from build123d import *

# Parameters (mm, degrees)
SKETCH1_R           = 3.429
SKETCH1_R_2         = 2.54
BOSS_EXTRUDE1_DEPTH = 3.2004
SKETCH2_R           = 2.413
CUT_EXTRUDE1_DEPTH  = 3.2004
SKETCH5_R           = 1.7272
SKETCH5_W           = 40.894
SKETCH5_H           = 20.32
CUT_EXTRUDE3_DEPTH  = 203.721029268
CUT_EXTRUDE5_DEPTH  = 3.2004
SKETCH6_R           = 2.54
CUT_EXTRUDE4_DEPTH  = 203.721029268
SKETCH9_R           = 2.159
CUT_EXTRUDE6_DEPTH  = 3.2004
SKETCH10_W          = 107.95
SKETCH10_H          = 3.2512
CUT_EXTRUDE7_DEPTH  = 3.2004
SKETCH11_R          = 3.429
SKETCH11_R_2        = 2.54
CUT_EXTRUDE8_DEPTH  = 3.2004
CUT_EXTRUDE9_DEPTH  = 3.2004
SKETCH15_R          = 2.159
CUT_EXTRUDE10_DEPTH = 3.2004
BOSS_EXTRUDE2_DEPTH = 3.2004
FILLET1_R           = 5.08
CUT_EXTRUDE11_DEPTH = 3.2004
CUT_EXTRUDE12_DEPTH = 3.2004
FILLET3_R           = 5.08


with BuildPart() as part:
    # Sketch1 → Boss-Extrude1 (new body)
    with BuildSketch(Plane.XY):
        with BuildLine():
            Line((0, 0), (120.015, 0))
            ThreePointArc((120.015, 0), (130.351788396, 3.075697789), (137.325636158, 11.302152592))
            Line((137.325636158, 11.302152592), (155.2575, 52.11572))
            ThreePointArc((155.2575, 52.11572), (157.54731739, 67.602183396), (151.630955452, 82.09599151))
            ThreePointArc((151.630955452, 82.09599151), (60.0075, 127.266502568), (-31.615955452, 82.09599151))
            ThreePointArc((-31.615955452, 82.09599151), (-37.53231739, 67.602183396), (-35.2425, 52.11572))
            Line((-35.2425, 52.11572), (-17.310636158, 11.302152592))
            ThreePointArc((-17.310636158, 11.302152592), (-10.336788396, 3.075697789), (0, 0))
        make_face()
        with Locations((120.015, 18.90776)):
            Circle(SKETCH1_R, mode=Mode.SUBTRACT)
        with Locations((0, 18.90776)):
            Circle(SKETCH1_R_2, mode=Mode.SUBTRACT)
        with Locations((19.734727626, 25.566426992)):
            Circle(SKETCH1_R_2, mode=Mode.SUBTRACT)
    extrude(amount=BOSS_EXTRUDE1_DEPTH)

    # Sketch2 → Cut-Extrude1 (cut)
    with BuildSketch(Plane(origin=(0, 0, 0), x_dir=(-1, 0, 0), z_dir=(0, 0, -1))):
        with Locations((-92.0115, 52.11572)):
            Circle(SKETCH2_R)
        with Locations((-76.0095, 52.11572)):
            Circle(SKETCH2_R)
        with Locations((-44.0055, 52.11572)):
            Circle(SKETCH2_R)
        with Locations((-28.0035, 52.11572)):
            Circle(SKETCH2_R)
    extrude(amount=-CUT_EXTRUDE1_DEPTH, mode=Mode.SUBTRACT)

    # Sketch5 → Cut-Extrude3 (cut, through all)
    with BuildSketch(Plane(origin=(0, 0, 0), x_dir=(-1, 0, 0), z_dir=(0, 0, -1))):
        with Locations((-98.932021353, 23.907759967)):
            Circle(SKETCH5_R)
        with Locations((-48.432021353, 13.907760033)):
            Circle(SKETCH5_R)
        with Locations((-48.432021353, 23.907759967)):
            Circle(SKETCH5_R)
        with Locations((-98.932021353, 13.907760033)):
            Circle(SKETCH5_R)
        with Locations((-73.682021353, 18.90776)):
            Rectangle(SKETCH5_W, SKETCH5_H)
    extrude(amount=-CUT_EXTRUDE3_DEPTH, mode=Mode.SUBTRACT)

    # Sketch7 → Cut-Extrude5 (cut)
    with BuildSketch(Plane(origin=(0, 0, 0), x_dir=(-1, 0, 0), z_dir=(0, 0, -1))):
        with BuildLine():
            Line((-98.193021353, 19.92376), (-94.129021353, 19.92376))
            Line((-94.129021353, 19.92376), (-94.129021353, 17.89176))
            Line((-94.129021353, 17.89176), (-98.193021353, 17.89176))
            ThreePointArc((-98.193021353, 17.89176), (-99.209021353, 18.90776), (-98.193021353, 19.92376))
        make_face()
        with BuildLine():
            Line((-53.235021353, 19.92376), (-49.171021353, 19.92376))
            ThreePointArc((-49.171021353, 19.92376), (-48.155021353, 18.90776), (-49.171021353, 17.89176))
            Line((-49.171021353, 17.89176), (-53.235021353, 17.89176))
            Line((-53.235021353, 17.89176), (-53.235021353, 19.92376))
        make_face()
    extrude(amount=-CUT_EXTRUDE5_DEPTH, mode=Mode.SUBTRACT)

    # Sketch6 → Cut-Extrude4 (cut, through all)
    with BuildSketch(Plane(origin=(0, 0, 0), x_dir=(-1, 0, 0), z_dir=(0, 0, -1))):
        with Locations((-99.400822485, 30.809360937)):
            Circle(SKETCH6_R)
    extrude(amount=-CUT_EXTRUDE4_DEPTH, mode=Mode.SUBTRACT)

    # Sketch9 → Cut-Extrude6 (cut)
    with BuildSketch(Plane.XY.offset(3.2004)):
        with Locations((21.9075, 3.81)):
            Circle(SKETCH9_R)
        with Locations((60.0075, 3.81)):
            Circle(SKETCH9_R)
        with Locations((98.1075, 3.81)):
            Circle(SKETCH9_R)
    extrude(amount=-CUT_EXTRUDE6_DEPTH, mode=Mode.SUBTRACT)

    # Sketch10 → Cut-Extrude7 (cut)
    with BuildSketch(Plane.XY.offset(3.2004)):
        with Locations((60.0075, 46.68012)):
            Rectangle(SKETCH10_W, SKETCH10_H)
    extrude(amount=-CUT_EXTRUDE7_DEPTH, mode=Mode.SUBTRACT)

    # Sketch11 → Cut-Extrude8 (cut)
    with BuildSketch(Plane.XY.offset(3.2004)):
        with Locations((126.474462556, 80.535782848)):
            Circle(SKETCH11_R)
        with Locations((105.860285087, 92.437383759)):
            Circle(SKETCH11_R_2)
    extrude(amount=-CUT_EXTRUDE8_DEPTH, mode=Mode.SUBTRACT)

    # Sketch14 → Cut-Extrude9 (cut)
    with BuildSketch(Plane(origin=(0, 0, 0), x_dir=(-1, 0, 0), z_dir=(0, 0, -1))):
        with BuildLine():
            Line((-44.300963253, 126.193661773), (-33.172711709, 93.735154568))
            Line((-33.172711709, 93.735154568), (17.974883496, 60.568226691))
            Line((17.974883496, 60.568226691), (31.788532543, 81.870619617))
            ThreePointArc((31.788532543, 81.870619617), (-1.866863458, 111.567353903), (-44.300963253, 126.193661773))
        make_face()
    extrude(amount=-CUT_EXTRUDE9_DEPTH, mode=Mode.SUBTRACT)

    # Sketch15 → Cut-Extrude10 (cut)
    with BuildSketch(Plane.XY.offset(3.2004)):
        with Locations((8.255, 18.90776)):
            Circle(SKETCH15_R)
        with Locations((107.05592, 18.90776)):
            Circle(SKETCH15_R)
    extrude(amount=-CUT_EXTRUDE10_DEPTH, mode=Mode.SUBTRACT)

    # Sketch16 → Boss-Extrude2 (add)
    with BuildSketch(Plane.XY.offset(3.2004)):
        with BuildLine():
            Line((-45.041102147, 54.757414103), (-19.827237301, 11.4051976))
            ThreePointArc((-19.827237301, 11.4051976), (-11.436759498, 3.05471175), (0, 0))
            ThreePointArc((0, 0), (-10.916945649, 29.711492853), (-17.974883496, 60.568226691))
            Line((-17.974883496, 60.568226691), (-35.838426308, 88.116067724))
            ThreePointArc((-35.838426308, 88.116067724), (-39.004683679, 85.006183785), (-42.068546328, 81.795372437))
            ThreePointArc((-42.068546328, 81.795372437), (-48.007013112, 68.765867356), (-45.041102147, 54.757414103))
        make_face()
    extrude(amount=-BOSS_EXTRUDE2_DEPTH)

    # Fillet1
    fillet1_edges = [part.edges().sort_by_distance(p)[0] for p in [
        (44.300963253, 126.193661773, 1.6002),
        (-35.838426308, 88.116067724, 1.6002),
    ]]
    fillet(fillet1_edges, radius=FILLET1_R)

    # Sketch17 → Cut-Extrude11 (cut)
    with BuildSketch(Plane(origin=(0, 0, 0), x_dir=(-1, 0, 0), z_dir=(0, 0, -1))):
        with BuildLine():
            Line((-34.3535, 67.35572), (-21.6535, 67.35572))
            ThreePointArc((-21.6535, 67.35572), (-18.4785, 64.18072), (-21.6535, 61.00572))
            Line((-21.6535, 61.00572), (-34.3535, 61.00572))
            ThreePointArc((-34.3535, 61.00572), (-37.5285, 64.18072), (-34.3535, 67.35572))
        make_face()
    extrude(amount=-CUT_EXTRUDE11_DEPTH, mode=Mode.SUBTRACT)

    # Sketch18 → Cut-Extrude12 (cut)
    with BuildSketch(Plane(origin=(0, 0, 0), x_dir=(-1, 0, 0), z_dir=(0, 0, -1))):
        Polygon((39.398034495, 93.605433495), (17.974883496, 60.568226691), (70.53521478, 66.420124121), align=None)
    extrude(amount=-CUT_EXTRUDE12_DEPTH, mode=Mode.SUBTRACT)

    # Fillet3
    fillet3_edges = [part.edges().sort_by_distance(p)[0] for p in [
        (-48.023040183, 63.913691353, 1.6002),
    ]]
    fillet(fillet3_edges, radius=FILLET3_R)


solid = part.part
CAD build for the part. Positions are in the model's coordinates, mm. Round coordinates to 2 decimals unless told otherwise and drop trailing zeros. Write each loop counter-clockwise with the first axis right and the second up, starting at its lowest first coordinate (ties: lowest second). Pieces come first, ordered by that corner, then holes.
(1) Drop flat-ended pins along their axis: P1, Ø1, axis at x = 95.5, z = 1.5, coming from the +Y side; P2, Ø1, axis at y = 89.5, z = 1, coming from the -X side; P3, Ø1.5, axis at x = 130, z = 1.5, coming from the -Y side. Give the stop position or say it passes through.
(2) Slice it at B-B, the plane y = 3.81. Write the cut outline in (x, z).
(3) Mould opens along Y. For faces 1 (the face through (77, 65, 0)), 2 (the face through (100.167, 4.459, 1.623)), 3 (the face through (38.292, 108.668, 1.578)), 4 (the face through (146.166, 31.423, 1.578)) say: pulls with the +Y half, pulls with the -Y half, needs draft (parallel to the pull), parting line crosses it, or undercut.
(4) Probe line 1 along Y through (x, z) = (21.5, 1.15); line 2 along Y through (x, z) = (49, 2.8); line 3 along Y through (x, z) = (88.5, 2.45). List the from-to ranges inside material, lowest first.
(5) Slice it at C-C, the plane y = 40. Write the cut outline in (x, z), and give its area (3 significant figures).
(6) Slice it at A-A, the plane x = 66.5. Write the cut outline in (y, z), and give its area (3 significant figures).
(7) Slice it at D-D, the plane z = 2. Count the separate pieces of the cut face and the enclosed holes in it, and give its area (3 significant figures).
From the geometry:
1. P1: stops at y = 121.84
1. P2: stops at x = 25.87
1. P3: stops at y = 2.41
2. outline: (-12.66, 0) - (19.75, 0) - (19.75, 3.2) - (-12.66, 3.2) - close; (24.07, 0) - (57.85, 0) - (57.85, 3.2) - (24.07, 3.2) - close; (62.17, 0) - (95.95, 0) - (95.95, 3.2) - (62.17, 3.2) - close; (100.27, 0) - (131.4, 0) - (131.4, 3.2) - (100.27, 3.2) - close
3. face 1: needs draft
3. face 2: undercut
3. face 3: pulls with the +Y half
3. face 4: pulls with the -Y half
4. line 1: y = 0 to 1.69, 5.93 to 23.74, 27.39 to 45.05, 48.31 to 61.01, 67.35 to 86.17
4. line 2: y = 0 to 12.28, 15.54 to 17.91, 19.91 to 22.28, 25.54 to 45.05, 48.31 to 126.74
4. line 3: y = 0 to 8.75, 29.07 to 45.05, 48.31 to 123.7
5. outline: (-36.46, 0) - (149.93, 0) - (149.93, 3.2) - (-36.46, 3.2) - close
5. area: 597 mm2
6. outline: (0, 0) - (8.75, 0) - (8.75, 3.2) - (0, 3.2) - close; (29.07, 0) - (45.05, 0) - (45.05, 3.2) - (29.07, 3.2) - close; (48.31, 0) - (127.08, 0) - (127.08, 3.2) - (48.31, 3.2) - close
6. area: 331 mm2
7. separate pieces: 1
7. enclosed holes: 22
7. area: 16,400 mm2
